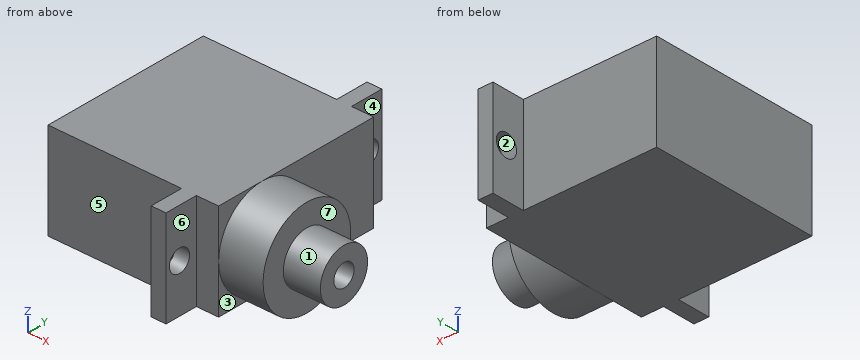
from build123d import *

# Parameters (mm, degrees)
CYLINDER010_R          = 1.5
CYLINDER010_DEPTH      = 10
CYLINDER013_R          = 1.5
CYLINDER013_DEPTH      = 5
CYLINDER014_R          = 1.5
CYLINDER014_DEPTH      = 10
CYLINDER011_R          = 3.5
CYLINDER011_DEPTH      = 5
BOX004_W               = 32
BOX004_H               = 13
BOX004_DEPTH           = 2
CYLINDER012_R          = 6.5
CYLINDER012_DEPTH      = 6
BOX005_W               = 23
BOX005_H               = 13
BOX005_DEPTH           = 23
CUT002_ROLL_ANGLE      = -90
CUT002_PLACEMENT_ANGLE = -90


with BuildPart() as zylinder010:
    # Cylinder010 → Cylinder010 (new body)
    with BuildSketch(Plane(origin=(25.5, 6.5, 13), x_dir=(1, 0, 0), z_dir=(0, 0, 1))):
        Circle(CYLINDER010_R)
    extrude(amount=CYLINDER010_DEPTH)


with BuildPart() as zylinder013:
    # Cylinder013 → Cylinder013 (new body)
    with BuildSketch(Plane(origin=(16.5, 6.5, 30), x_dir=(1, 0, 0), z_dir=(0, 0, 1))):
        Circle(CYLINDER013_R)
    extrude(amount=CYLINDER013_DEPTH)


with BuildPart() as fusion004:
    # Cylinder014 → Cylinder014 (new body)
    with BuildSketch(Plane(origin=(-2.5, 6.5, 13), x_dir=(1, 0, 0), z_dir=(0, 0, 1))):
        Circle(CYLINDER014_R)
    extrude(amount=CYLINDER014_DEPTH)

    # Fusion004: union Zylinder010, Zylinder013
    add(zylinder010.part)
    add(zylinder013.part)


with BuildPart() as zylinder011:
    # Cylinder011 → Cylinder011 (new body)
    with BuildSketch(Plane(origin=(16.5, 6.5, 29), x_dir=(1, 0, 0), z_dir=(0, 0, 1))):
        Circle(CYLINDER011_R)
    extrude(amount=CYLINDER011_DEPTH)


with BuildPart() as obj1:
    # Box004 → Box004 (new body)
    with BuildSketch(Plane(origin=(-4.5, 0, 18), x_dir=(1, 0, 0), z_dir=(0, 0, 1))):
        with Locations((16, 6.5)):
            Rectangle(BOX004_W, BOX004_H)
    extrude(amount=BOX004_DEPTH)


with BuildPart() as zylinder012:
    # Cylinder012 → Cylinder012 (new body)
    with BuildSketch(Plane(origin=(16.5, 6.5, 23), x_dir=(1, 0, 0), z_dir=(0, 0, 1))):
        Circle(CYLINDER012_R)
    extrude(amount=CYLINDER012_DEPTH)


with BuildPart() as servo3:
    # Box005 → Box005 (new body)
    with BuildSketch(Plane.XY):
        with Locations((11.5, 6.5)):
            Rectangle(BOX005_W, BOX005_H)
    extrude(amount=BOX005_DEPTH)

    # Fusion005: union Zylinder011, obj1, Zylinder012
    add(zylinder011.part)
    add(obj1.part)
    add(zylinder012.part)

    # Cut002: cut Fusion004
    add(fusion004.part, mode=Mode.SUBTRACT)


with BuildPart() as servo3_1:
    # Cut002 roll: moved
    add(servo3.part.rotate(Axis((0, 0, 0), (1, 0, 0)), CUT002_ROLL_ANGLE))


with BuildPart() as servo3_2:
    # Cut002 placement: moved
    add(servo3_1.part.moved(Location((-49.5, 16.5, 6))).rotate(Axis((-49.5, 16.5, 6), (0, 0, 1)), CUT002_PLACEMENT_ANGLE))


solid = servo3_2.part
Here's how the part is built. I have some questions about the finished solid (model axes, mm). Face numbers are marked on the shaded views. A direction names the side the tool comes from. Give positions to 0.01 mm unless a question says otherwise; leave off trailing zeros. Order: outer loops, then holes, each group sorted by start corner. A loop starts at its lowest first (then second) coordinate and runs counter-clockwise, first axis right, second up. Notation, with made-up numbers: M -15,-34 L 22,-34 A33 ccw 22,-4 Z; hole C -10,48.5 d5. An arc over 180 degrees is marked long. Answer as a JSON object with one key per item and string values. Group by question number.
1) Suppose I cut it at C-C, the plane x = -41. Write out the boundary of the cut face in (y, z), plus the area to 3 significant figures.
2) I'm going to push flat-ended pins straight in: pin 1 Ø6.5 at (x, z) = (-38, -1) entering from +Y; pin 2 Ø3 at (y, z) = (-2.5, -5) entering from +X; pin 3 Ø1 at (y, z) = (11.5, 0.5) entering from +X. Where does each tip first touch, or does it pass through?
3) We'd pull the mould along Y, two halves only. Please class the marked faces 1, 2 and 3: pulls with the +Y half, pulls with the -Y half, needs draft (parallel to the pull), parting line crosses it, or undercut.
4) Suppose I cut it at B-B, the plane z = 0.25. Count the separate pieces of the cut face and the enclosed holes in it, plus the area to 3 significant figures.
5) Suppose I cut it at D-D, the plane z = -5. Write out the boundary of the cut face in (x, y).
6) Please list where these lines run through material, in increasing order: L1, parallel to Z at x = -18.45, y = 0; L2, parallel to Y at x = -33.5, z = -2.5; L3, parallel to X at y = -5, z = -6. Write a range as [from, to].
7) Suppose I cut it at A-A, the plane y = 19. Write out the boundary of the cut face in (x, z), plus the area to 3 significant figures.
8) On a 3-axis mill with a long thin cutter (end or side, diameter ignored), from which of +Z, -Z, +X, -X, +Y, -Y can I reach the whole of each face in a straight line? I mean the marked faces 4, 5, 6 and 7. Say none if no direction works.
Results found:
{
 "1": {"outline": "M -6.5,-7 L 16.5,-7 L 16.5,6 L -6.5,6 Z", "area": "299 mm²"},
 "2": {"pin 1": "y = 16.5", "pin 2": "x = -20.5", "pin 3": "x = -26.5"},
 "3": {"face 1": "parting line crosses it", "face 2": "undercut", "face 3": "needs draft"},
 "4": {"separate pieces": "3", "enclosed holes": "0", "area": "638 mm²"},
 "5": {"outline": "M -49.5,-6.5 L -31.5,-6.5 L -31.5,-11 L -29.5,-11 L -29.5,-6.5 L -26.5,-6.5 L -26.5,-4.69 L -20.5,-4.69 L -20.5,4.69 L -26.5,4.69 L -26.5,16.5 L -29.5,16.5 L -29.5,21 L -31.5,21 L -31.5,16.5 L -49.5,16.5 Z"},
 "6": {"L1": "[-4, -2], [1, 3]", "L2": "[-6.5, 16.5]", "L3": "[-49.5, -26.5]"},
 "7": {"outline": "M -31.5,-7 L -29.5,-7 L -29.5,-2 L -31.5,-2 Z; M -31.5,1 L -29.5,1 L -29.5,6 L -31.5,6 Z", "area": "20.0 mm²"},
 "8": {"face 4": "+Z, -Z, +X, +Y", "face 5": "+Z, -Z, -X, -Y", "face 6": "+Z, -Z, +X, -Y", "face 7": "+X"}
}
